Could you check a few things on this model? Use its own coordinates, in mm. A direction names the side the tool comes from. Coordinates: 2 decimals unless noted, no trailing zeros. One line per question, with ' | ' between items.
from build123d import *

# Parameters (mm, degrees)
CROQUIS2_W                   = 220
CROQUIS2_H                   = 220
CROQUIS2_W_2                 = 200
CROQUIS2_H_2                 = 200
SALIENTE_EXTRUIR1_DEPTH      = 10
CROQUIS3_W                   = 212
CROQUIS3_H                   = 212
CROQUIS3_W_2                 = 210
CROQUIS3_H_2                 = 210
CROQUIS3_W_3                 = 208
CROQUIS3_H_3                 = 208
CORTAR_EXTRUIR1_DEPTH        = 3.5
CROQUIS4_W                   = 10
CROQUIS4_H                   = 10
SALIENTE_EXTRUIR2_DEPTH      = 200
SALIENTE_EXTRUIR2_DEPTH_BACK = 10
CROQUIS6_W                   = 3.5
CROQUIS6_H                   = 2
CROQUIS6_W_2                 = 2
CROQUIS6_H_2                 = 3.5
CROQUIS6_W_3                 = 1.99805467
CORTAR_EXTRUIR2_DEPTH        = 203.5
CROQUIS7_W                   = 220
CROQUIS7_H                   = 220
CROQUIS7_W_2                 = 200
CROQUIS7_H_2                 = 200
SALIENTE_EXTRUIR3_DEPTH      = 10
CORTAR_EXTRUIR3_START        = -3.5
CROQUIS8_W                   = 207
CROQUIS8_H                   = 2
CORTAR_EXTRUIR3_DEPTH        = 207
MATRIZC1_COUNT               = 4
CROQUIS9_W                   = 86
CROQUIS9_H                   = 16
BRAZOS_DEPTH                 = 10
MATRIZC2_COUNT               = 4


with BuildPart() as part:
    # Croquis2 → Saliente-Extruir1 (new body)
    with BuildSketch(Plane.XY):
        with Locations((110, -110)):
            Rectangle(CROQUIS2_W, CROQUIS2_H)
        with Locations((110, -110)):
            Rectangle(CROQUIS2_W_2, CROQUIS2_H_2, mode=Mode.SUBTRACT)
    extrude(amount=SALIENTE_EXTRUIR1_DEPTH)

    # Croquis3 → Cortar-Extruir1 (cut)
    with BuildSketch(Plane.XY.offset(10)):
        with Locations((110, -110)):
            Rectangle(CROQUIS3_W, CROQUIS3_H)
        with Locations((110, -110)):
            Rectangle(CROQUIS3_W_2, CROQUIS3_H_2, mode=Mode.SUBTRACT)
        with Locations((110, -110)):
            Rectangle(CROQUIS3_W_2, CROQUIS3_H_2)
        with Locations((110, -110)):
            Rectangle(CROQUIS3_W_3, CROQUIS3_H_3, mode=Mode.SUBTRACT)
    extrude(amount=-CORTAR_EXTRUIR1_DEPTH, mode=Mode.SUBTRACT)

    # Croquis4 → Saliente-Extruir2 (add, two sides)
    with BuildSketch(Plane.XY.offset(10)) as saliente_extruir2_sk:
        with Locations((5, -5)):
            Rectangle(CROQUIS4_W, CROQUIS4_H)
        with Locations((215, -5)):
            Rectangle(CROQUIS4_W, CROQUIS4_H)
        with Locations((215, -215)):
            Rectangle(CROQUIS4_W, CROQUIS4_H)
        with Locations((5, -215)):
            Rectangle(CROQUIS4_W, CROQUIS4_H)
    extrude(amount=SALIENTE_EXTRUIR2_DEPTH)
    extrude(saliente_extruir2_sk.sketch, amount=-SALIENTE_EXTRUIR2_DEPTH_BACK)

    # Croquis6 → Cortar-Extruir2 (cut)
    with BuildSketch(Plane.XY.offset(210)):
        with Locations((8.25, -5)):
            Rectangle(CROQUIS6_W, CROQUIS6_H)
        with Locations((5, -8.25)):
            Rectangle(CROQUIS6_W_2, CROQUIS6_H_2)
        with Locations((211.75, -5)):
            Rectangle(CROQUIS6_W, CROQUIS6_H)
        with Locations((215, -8.25)):
            Rectangle(CROQUIS6_W_2, CROQUIS6_H_2)
        with Locations((211.75, -215)):
            Rectangle(CROQUIS6_W, CROQUIS6_H)
        with Locations((215.000972665, -211.75)):
            Rectangle(CROQUIS6_W_3, CROQUIS6_H_2)
        with Locations((5, -211.75)):
            Rectangle(CROQUIS6_W_2, CROQUIS6_H_2)
        with Locations((8.25, -215)):
            Rectangle(CROQUIS6_W, CROQUIS6_H)
    extrude(amount=-CORTAR_EXTRUIR2_DEPTH, mode=Mode.SUBTRACT)

    # Croquis7 → Saliente-Extruir3 (add)
    with BuildSketch(Plane.XY.offset(210)):
        with Locations((110, -110)):
            Rectangle(CROQUIS7_W, CROQUIS7_H)
        with Locations((110, -110)):
            Rectangle(CROQUIS7_W_2, CROQUIS7_H_2, mode=Mode.SUBTRACT)
    extrude(amount=SALIENTE_EXTRUIR3_DEPTH)

    # Croquis8 → Cortar-Extruir3 (cut)
    with BuildSketch(Plane(origin=(0, -210, 0), x_dir=(1, 0, 0), z_dir=(0, 1, 0)).offset(CORTAR_EXTRUIR3_START)):
        with Locations((110, -215)):
            Rectangle(CROQUIS8_W, CROQUIS8_H)
    cortar_extruir3 = extrude(amount=CORTAR_EXTRUIR3_DEPTH, mode=Mode.SUBTRACT)

    # MatrizC1: Cortar-Extruir3 ×4 about axis
    matrizc1_axis = Axis((0, -110, 110), (1, 0, 0))
    for i in range(1, MATRIZC1_COUNT):
        add(cortar_extruir3.rotate(matrizc1_axis, i * 360 / MATRIZC1_COUNT), mode=Mode.SUBTRACT)

    # Croquis9 → Brazos (add)
    with BuildSketch(Plane.XY.offset(220)):
        with Locations((43, -110)):
            Rectangle(CROQUIS9_W, CROQUIS9_H)
        with BuildLine():
            ThreePointArc((71.801526277, -112.25), (69.551526277, -110), (71.801526277, -107.75))
            Line((71.801526277, -107.75), (75, -107.75))
            ThreePointArc((75, -107.75), (77.25, -110), (75, -112.25))
            Line((75, -112.25), (71.801526277, -112.25))
        make_face(mode=Mode.SUBTRACT)
        with Locations((177, -110)):
            Rectangle(CROQUIS9_W, CROQUIS9_H)
        with BuildLine():
            Line((145, -107.75), (148.198473723, -107.75))
            ThreePointArc((148.198473723, -107.75), (150.448473723, -110), (148.198473723, -112.25))
            Line((148.198473723, -112.25), (145, -112.25))
            ThreePointArc((145, -112.25), (142.75, -110), (145, -107.75))
        make_face(mode=Mode.SUBTRACT)
    extrude(amount=-BRAZOS_DEPTH)

    # MatrizC2: Cortar-Extruir3 ×4 about axis
    matrizc2_axis = Axis((110, 11, 110), (0, -1, 0))
    for i in range(1, MATRIZC2_COUNT):
        add(cortar_extruir3.rotate(matrizc2_axis, i * 360 / MATRIZC2_COUNT), mode=Mode.SUBTRACT)


solid = part.part
1) If we section it at A-A on z = 57: Give the number of separate pieces and of enclosed holes in the cut face, and give its area (3 significant figures).
Data:
separate pieces: 4 | enclosed holes: 0 | area: 344 mm²
2) I need wall thicknesses on line 1 along Y through (x, z) = (9, 142.5). Which ranges of the line are inside material? Lowest first, please. Write a range as from..to.
Data:
line 1: -220..-216, -214..-210, -10..-6, -4..0
3) We'd pull the mould along Y, two halves only. Please class faces 6 (the face through (9.85, -6, 156.48)), 7 (the face through (0, -119, 5)), 8 (the face through (101, 0, 215)): pulls with the +Y half, pulls with the -Y half, needs draft (parallel to the pull), parting line crosses it, or undercut.
Data:
face 6: undercut | face 7: needs draft | face 8: pulls with the +Y half
4) On a 3-axis mill with a long thin cutter (end or side, diameter ignored), from which of +Z, -Z, +X, -X, +Y, -Y can I reach the whole of each face in a straight line? I mean faces 1 (the face through (101, -215, 0)), 2 (the face through (216, -156.48, 210.15)), 3 (the face through (86, -110, 215)), 4 (the face through (37, -110, 210)), 5 (the face through (101, -220, 215)). Say none if no direction works.
Data:
face 1: -Z, +X, -X, +Y, -Y | face 2: none | face 3: +Z, -Z | face 4: +X, -X | face 5: +Z, -Z, +X, -X, -Y
